Geometry check sheet. Reference: the model listing, model coordinates, mm. Give positions to 0.01 mm unless a question says otherwise; leave off trailing zeros. Order: outer loops, then holes, each group sorted by start corner. A loop starts at its lowest first (then second) coordinate and runs counter-clockwise, first axis right, second up.
```python
from build123d import *

# Parameters (mm, degrees)
SKETCH5_R            = 2.794
BOSS_EXTRUDE21_DEPTH = 6.35
SKETCH6_R            = 2.794
CUT_EXTRUDE3_DEPTH   = 6.35
SKETCH7_R            = 5.08
CUT_EXTRUDE4_DEPTH   = 3.175


with BuildPart() as part:
    # Sketch5 → Boss-Extrude21 (new body)
    # profile 1 of 3: a face of its own
    with BuildSketch(Plane(origin=(0, 0, 0), x_dir=(1, 0, 0), z_dir=(0, 1, 0))):
        with BuildLine():
            Line((101.6, 12.7), (18.137479686, 12.7))
            Line((18.137479686, 12.7), (11.934096284, -4.34365582))
            ThreePointArc((11.934096284, -4.34365582), (7.284420742, -10.403230962), (0, -12.7))
            Line((0, -12.7), (101.6, -12.7))
            ThreePointArc((101.6, -12.7), (114.3, 0), (101.6, 12.7))
        make_face()
    # profile 2 of 3: a face of its own
    with BuildSketch(Plane(origin=(0, 0, 0), x_dir=(1, 0, 0), z_dir=(0, 1, 0))):
        with BuildLine():
            ThreePointArc((-11.934096284, 4.34365582), (-7.284420742, 10.403230962), (0, 12.7))
            Line((0, 12.7), (18.137479686, 12.7))
            Line((18.137479686, 12.7), (46.683342846, 91.129114452))
            ThreePointArc((46.683342846, 91.129114452), (39.092902382, 107.406866556), (22.815150278, 99.816426092))
            Line((22.815150278, 99.816426092), (-11.934096284, 4.34365582))
        make_face()
    # profile 3 of 3: a face of its own
    with BuildSketch(Plane(origin=(0, 0, 0), x_dir=(1, 0, 0), z_dir=(0, 1, 0))):
        with BuildLine():
            Line((18.137479686, 12.7), (0, 12.7))
            ThreePointArc((0, 12.7), (-7.284420742, 10.403230962), (-11.934096284, 4.34365582))
            ThreePointArc((-11.934096284, 4.34365582), (-10.403230962, -7.284420742), (0, -12.7))
            ThreePointArc((0, -12.7), (7.284420742, -10.403230962), (11.934096284, -4.34365582))
            Line((11.934096284, -4.34365582), (18.137479686, 12.7))
        make_face()
        with Locations(Location((0, 0, 0), (0, 0, 270))):
            Circle(SKETCH5_R, mode=Mode.SUBTRACT)
    extrude(amount=BOSS_EXTRUDE21_DEPTH)

    # Sketch6 → Cut-Extrude3 (cut)
    with BuildSketch(Plane(origin=(0, 0, 0), x_dir=(-1, 0, 0), z_dir=(0, -1, 0))):
        with Locations(Location((-50.8, 0, 0), (0, 0, 90))):
            Circle(SKETCH6_R)
        with Locations(Location((-17.374623281, 47.736385136, 0), (0, 0, 90))):
            Circle(SKETCH6_R)
        with Locations(Location((-25.4, 0, 0), (0, 0, 90))):
            Circle(SKETCH6_R)
        with Locations(Location((-76.2, 0, 0), (0, 0, 90))):
            Circle(SKETCH6_R)
        with Locations(Location((-8.68731164, 23.868192568, 0), (0, 0, 90))):
            Circle(SKETCH6_R)
        with Locations(Location((-26.061934921, 71.604577704, 0), (0, 0, 90))):
            Circle(SKETCH6_R)
    extrude(amount=-CUT_EXTRUDE3_DEPTH, mode=Mode.SUBTRACT)

    # Sketch7 → Cut-Extrude4 (cut)
    with BuildSketch(Plane(origin=(0, 6.35, 0), x_dir=(1, 0, 0), z_dir=(0, 1, 0))):
        with Locations(Location((26.061934921, 71.604577704, 0), (0, 0, 270))):
            Circle(SKETCH7_R)
        with Locations(Location((17.374623281, 47.736385136, 0), (0, 0, 270))):
            Circle(SKETCH7_R)
        with Locations(Location((8.68731164, 23.868192568, 0), (0, 0, 270))):
            Circle(SKETCH7_R)
        with Locations(Location((0, 0, 0), (0, 0, 270))):
            Circle(SKETCH7_R)
        with Locations(Location((25.4, 0, 0), (0, 0, 270))):
            Circle(SKETCH7_R)
        with Locations(Location((50.8, 0, 0), (0, 0, 270))):
            Circle(SKETCH7_R)
        with Locations(Location((76.2, 0, 0), (0, 0, 270))):
            Circle(SKETCH7_R)
    extrude(amount=-CUT_EXTRUDE4_DEPTH, mode=Mode.SUBTRACT)


solid = part.part
```
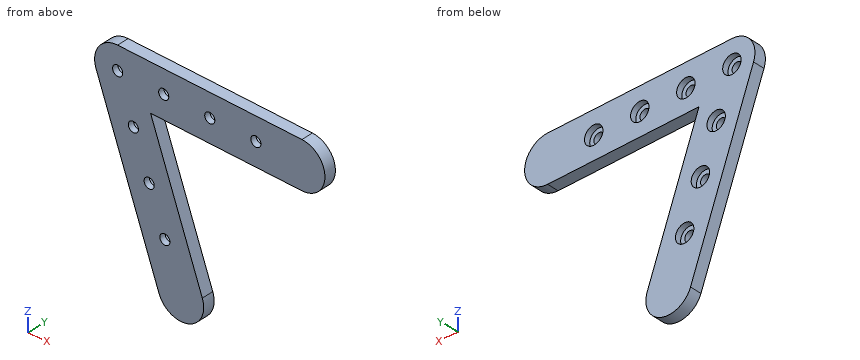
Q1. Cross-section at B-B, the plane y = 5. Record the boundary of the cut face in (x, z).
Q2. Cross-section at A-A, the plane x = 76.2. Record the boundary of the cut face in (y, z) (3 decimals), and give its area (3 significant figures).
Q3. Thickness scan on L1, parallel to X at y = 2.3, z = 0; L2, parallel to Z at x = 51, y = 1; L3, parallel to Z at x = 65.5, y = 0.75. Record the ranges inside material, lowest first.
Q4. Cross-section at C-C, the plane x = 98. Record the boundary of the cut face in (y, z), and give its area (3 significant figures).
Q5. Gauge pin test, flat ends, axial feed: P1, Ø3, axis at x = 18.5, z = -50.5, coming from the +Y side (3 decimals); P2, Ø8, axis at x = 26.06, z = -71.6, coming from the -Y side; P3, Ø1, axis at y = 5.5, z = -1, coming from the +X side; P4, Ø3, axis at y = 4, z = -17, coming from the +X side. Record the tip position at first contact, or that the pin passes through.
Q6. Cross-section at D-D, the plane z = 0. Give the number of separate pieces and of enclosed holes in the cut face, and give its area (3 significant figures).
Answers follow:
1. outline: (-11.93, -4.34) - (22.82, -99.82) arc R12.7 ccw to (46.68, -91.13) - (18.14, -12.7) - (101.6, -12.7) arc R12.7 ccw to (101.6, 12.7) - (0, 12.7) arc R12.7 ccw to start; hole circle Ø10.16 at (0, 0); hole circle Ø10.16 at (8.69, -23.87); hole circle Ø10.16 at (17.37, -47.74); hole circle Ø10.16 at (25.4, 0); hole circle Ø10.16 at (26.06, -71.6); hole circle Ø10.16 at (50.8, 0); hole circle Ø10.16 at (76.2, 0)
2. outline: (0, -12.7) - (6.35, -12.7) - (6.35, -5.08) - (3.175, -5.08) - (3.175, -2.794) - (0, -2.794) - close; (0, 2.794) - (3.175, 2.794) - (3.175, 5.08) - (6.35, 5.08) - (6.35, 12.7) - (0, 12.7) - close
2. area: 111 mm2
3. L1: x = -12.7 to -2.79, 2.79 to 22.61, 28.19 to 48.01, 53.59 to 73.41, 78.99 to 114.3
3. L2: z = -12.7 to -2.79, 2.79 to 12.7
3. L3: z = -12.7 to 12.7
4. outline: (0, -12.7) - (6.35, -12.7) - (6.35, 12.7) - (0, 12.7) - close
4. area: 161 mm2
5. P1: stops at y = 3.175
5. P2: stops at y = 0
5. P3: stops at x = 114.29
5. P4: stops at x = 20.25
6. separate pieces: 5
6. enclosed holes: 0
6. area: 606 mm2
